Source: CAD feature listing. Evaluate the final solid. Frame: model axes, mm. A direction names the side the tool comes from. Give positions to 0.01 mm unless a question says otherwise; leave off trailing zeros. Order: outer loops, then holes, each group sorted by start corner. A loop starts at its lowest first (then second) coordinate and runs counter-clockwise, first axis right, second up.
```python
from build123d import *

# Parameters (mm, degrees)
BOSS_EXTRU_1_DEPTH      = 9
BOSS_EXTRU_2_DEPTH      = 2
CONG_1_R                = 3
CONG_2_R                = 3
ENL_V_MAT_EXTRU_2_DEPTH = 1.2
ENL_V_MAT_EXTRU_3_DEPTH = 0.9
BOSS_EXTRU_3_DEPTH      = 2
ESQUISSE9_W             = 60
ESQUISSE9_H             = 2
BOSS_EXTRU_4_DEPTH      = 34
BOSS_EXTRU_5_DEPTH      = 3


with BuildPart() as part:
    # Esquisse1 → Boss.-Extru.1 (new body)
    with BuildSketch(Plane.XY):
        Polygon((-75, 41.958994513), (-30.446686156, 106.182331026), (30.446686156, 106.182331026), (75, 41.958994513), (75, -54.666809259), (-75, -54.666809259), align=None)
        Polygon((73, -52.666809259), (-73, -52.666809259), (-73, 41.333190741), (-29.4, 104.182331026), (29.4, 104.182331026), (73, 41.333190741), align=None, mode=Mode.SUBTRACT)
    extrude(amount=-BOSS_EXTRU_1_DEPTH)

    # Esquisse2 → Boss.-Extru.2 (add)
    with BuildSketch(Plane.XY):
        Polygon((-73, 41.333190741), (-29.4, 104.182331026), (29.4, 104.182331026), (73, 41.333190741), (73, -52.666809259), (-73, -52.666809259), align=None)
    extrude(amount=-BOSS_EXTRU_2_DEPTH)

    # Congé1
    cong_1_edges = [part.edges().sort_by_distance(p)[0] for p in [
        (29.4, 104.182331026, -5.5),
        (73, 41.333190741, -5.5),
        (73, -52.666809259, -5.5),
        (-73, -52.666809259, -5.5),
        (-73, 41.333190741, -5.5),
        (-29.4, 104.182331026, -5.5),
    ]]
    fillet(cong_1_edges, radius=CONG_1_R)

    # Congé2
    cong_2_edges = [part.edges().sort_by_distance(p)[0] for p in [
        (-75, 41.958994513, -4.5),
        (-30.446686156, 106.182331026, -4.5),
        (30.446686156, 106.182331026, -4.5),
        (75, 41.958994513, -4.5),
        (75, -54.666809259, -4.5),
        (-75, -54.666809259, -4.5),
        (-52.723343078, 74.07066277, 0),
        (0, 106.182331026, 0),
        (52.723343078, 74.07066277, 0),
        (75, -6.353907373, 0),
        (0, -54.666809259, 0),
        (-75, -6.353907373, 0),
    ]]
    fillet(cong_2_edges, radius=CONG_2_R)

    # Esquisse3 → Enlèv. mat.-Extru.2 (cut)
    with BuildSketch(Plane.XY):
        with BuildLine():
            ThreePointArc((14.913911185, 63.744265219), (15.827091675, 62.73511926), (16.775234523, 61.75874878))
            ThreePointArc((16.775234523, 61.75874878), (31.162887196, 69.020353616), (30.632630303, 52.91276901))
            ThreePointArc((30.632630303, 52.91276901), (36.012189208, 51.35807643), (41.559939675, 50.597032557))
            ThreePointArc((41.559939675, 50.597032557), (34.810541761, 70.493663133), (14.913911185, 63.744265219))
        make_face()
        with BuildLine():
            ThreePointArc((-16.775234523, 61.75874878), (-15.827091675, 62.73511926), (-14.913911185, 63.744265219))
            ThreePointArc((-14.913911185, 63.744265219), (-34.810541761, 70.493663133), (-41.559939675, 50.597032557))
            ThreePointArc((-41.559939675, 50.597032557), (-36.012189208, 51.35807643), (-30.632630303, 52.91276901))
            ThreePointArc((-30.632630303, 52.91276901), (-31.162887196, 69.020353616), (-16.775234523, 61.75874878))
        make_face()
    extrude(amount=-ENL_V_MAT_EXTRU_2_DEPTH, mode=Mode.SUBTRACT)

    # Esquisse7 → Enlèv. mat.-Extru.3 (cut)
    with BuildSketch(Plane.XY):
        with BuildLine():
            ThreePointArc((-30.632630303, 52.91276901), (-31.162887196, 69.020353616), (-16.775234523, 61.75874878))
            ThreePointArc((-16.775234523, 61.75874878), (-23.08615551, 56.36799961), (-30.632630303, 52.91276901))
        make_face()
        with BuildLine():
            ThreePointArc((30.632630303, 52.91276901), (31.16562065, 69.024635625), (16.775234523, 61.75874878))
            ThreePointArc((16.775234523, 61.75874878), (23.08615551, 56.36799961), (30.632630303, 52.91276901))
        make_face()
    extrude(amount=-ENL_V_MAT_EXTRU_3_DEPTH, mode=Mode.SUBTRACT)

    # Esquisse8 → Boss.-Extru.3 (add)
    with BuildSketch(Plane.XY):
        with BuildLine():
            Line((-22, 7.097367508), (-32, 11.705065554))
            ThreePointArc((-32, 11.705065554), (-48.741759908, -9.507732006), (-52, -36.334084286))
            ThreePointArc((-52, -36.334084286), (-30.801710364, -18.899787662), (-22, 7.097367508))
        make_face()
        with BuildLine():
            Line((22, 7.097367508), (32, 11.705065554))
            ThreePointArc((32, 11.705065554), (48.741759908, -9.507732006), (52, -36.334084286))
            ThreePointArc((52, -36.334084286), (30.801710364, -18.899787662), (22, 7.097367508))
        make_face()
    extrude(amount=BOSS_EXTRU_3_DEPTH)

    # Esquisse9 → Boss.-Extru.4 (add)
    with BuildSketch(Plane(origin=(0, 0, -9), x_dir=(-1, 0, 0), z_dir=(0, 0, -1))):
        with Locations((0, -53.666809259)):
            Rectangle(ESQUISSE9_W, ESQUISSE9_H)
    extrude(amount=BOSS_EXTRU_4_DEPTH)

    # Esquisse10 → Boss.-Extru.5 (add)
    with BuildSketch(Plane(origin=(0, -52.666809259, 0), x_dir=(1, 0, 0), z_dir=(0, 1, 0))):
        with BuildLine():
            Line((25, 41), (-25, 41))
            ThreePointArc((-25, 41), (0, 16), (25, 41))
        make_face()
    extrude(amount=BOSS_EXTRU_5_DEPTH)


solid = part.part
```
1) Section query D-D, the plane y = -28. Return the cut outline in (x, z).
Report:
outline: (-75, -9) - (-73, -9) - (-73, -2) - (73, -2) - (73, -9) - (75, -9) - (75, -3) arc R3 ccw to (72, 0) - (52.58, 0) - (52.58, 2) - (38.89, 2) - (38.89, 0) - (-38.89, 0) - (-38.89, 2) - (-52.58, 2) - (-52.58, 0) - (-72, 0) arc R3 ccw to (-75, -3) - close
2) Draft query along X for faces 5 (the flat face through (-26, 62, -0.9)), 6 (the cylindrical face through (-51.899, 73.759, -0.902)), 7 (the flat face through (52.6, 74.25, -5.96)), 8 (the flat face through (0, -49.667, -31)). Return one class per face: +X half, -X half, draft (parallel to the pull), parting line (faces both ways), or undercut.
Report:
face 5: undercut
face 6: -X half
face 7: +X half
face 8: draft
3) Reachability of faces 1 (the flat face through (26.93, 9.37, 0.99)), 2 (the flat face through (26, 62, -0.9)), 3 (the cylindrical face through (-31.024, -19.219, 0.986)), 4 (the flat face through (0, 104.182, -5)) from +Z, -Z, +X, -X, +Y, -Y: full face, straight path, thin tool, end or side. Return the list, or none.
Report:
face 1: +Z, +Y
face 2: +Z
face 3: +Z, -Y
face 4: -Z
4) Section query B-B, the plane x = 0. Return the cut outline in (y, z).
Report:
outline: (-54.67, -43) - (-52.67, -43) - (-52.67, -41) - (-49.67, -41) - (-49.67, -16) - (-52.67, -16) - (-52.67, -2) - (104.18, -2) - (104.18, -9) - (106.18, -9) - (106.18, -3) arc R3 ccw to (103.18, 0) - (-51.67, 0) arc R3 ccw to (-54.67, -3) - close
5) Material intervals for L1, parallel to Y at x = 19, z = -38.5; L2, parallel to Z at x = -0.5, y = 63; L3, parallel to Z at x = 47, y = -16.5, sorted ascending.
Report:
L1: y = -54.67 to -49.67
L2: z = -2 to 0
L3: z = -2 to 2
6) Section query C-C, the plane z = -23.5. Return the cut outline in (x, y), and give its area (3 significant figures).
Report:
outline: (-30, -54.67) - (30, -54.67) - (30, -52.67) - (17.85, -52.67) - (17.85, -49.67) - (-17.85, -49.67) - (-17.85, -52.67) - (-30, -52.67) - close
area: 227 mm2
7) Section query A-A, the plane y = 28. Return the cut outline in (x, z).
Report:
outline: (-75, -9) - (-73, -9) - (-73, -2) - (73, -2) - (73, -9) - (75, -9) - (75, -3) arc R3 ccw to (72, 0) - (-72, 0) arc R3 ccw to (-75, -3) - close
8) Pin query (flat end, axial travel): pin 1 (6.5 mm diameter, centred on x = 22.5, y = 61, fed in from +Z); pin 2 (23.5 mm diameter, centred on x = -27.5, y = 63.5, fed in from +Z); pin 3 (1.6 mm diameter, centred on y = -53.5, z = -30.5, fed in from +X). Return the tip coordinate at first contact, or that it passes through.
Report:
pin 1: stops at z = -0.9
pin 2: stops at z = 0
pin 3: stops at x = 30
